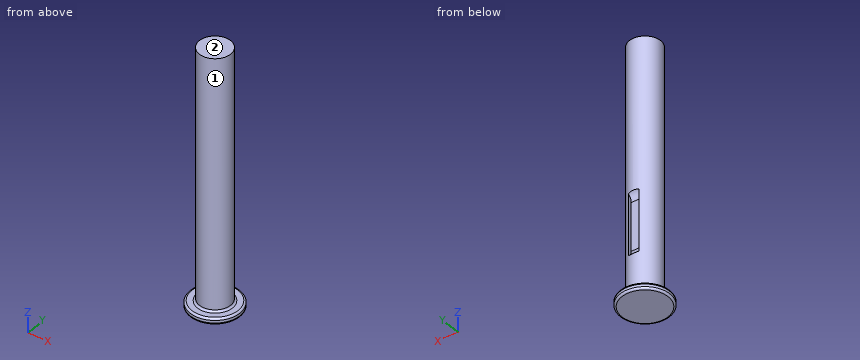
```python
from build123d import *

# Parameters (mm, degrees)
SKETCH1_R           = 8
BOSS_EXTRUDE1_DEPTH = 2
SKETCH2_R           = 5
BOSS_EXTRUDE2_DEPTH = 80
CUT_EXTRUDE1_DEPTH  = 1.75
FILLET2_R           = 0.6


with BuildPart() as part:
    # Sketch1 → Boss-Extrude1 (new body)
    with BuildSketch(Plane.XY):
        Circle(SKETCH1_R)
    extrude(amount=BOSS_EXTRUDE1_DEPTH)

    # Sketch2 → Boss-Extrude2 (add)
    with BuildSketch(Plane.XY.offset(2)):
        Circle(SKETCH2_R)
    extrude(amount=BOSS_EXTRUDE2_DEPTH)

    # Sketch4 → Cut-Extrude1 (cut, symmetric)
    with BuildSketch(Plane(origin=(0, 0, 0), x_dir=(0, 0, -1), z_dir=(1, 0, 0))):
        with BuildLine():
            Line((-34, 5), (-14, 5))
            ThreePointArc((-14, 5), (-14.921981454, 3.908349934), (-16.291287847, 3.5))
            Line((-16.291287847, 3.5), (-31.708712153, 3.5))
            ThreePointArc((-31.708712153, 3.5), (-33.078018546, 3.908349934), (-34, 5))
        make_face()
    extrude(amount=CUT_EXTRUDE1_DEPTH, both=True, mode=Mode.SUBTRACT)

    # Fillet2
    fillet2_edges = [part.edges().sort_by_distance(p)[0] for p in [
        (-8, 0, 0),
        (-8, 0, 2),
        (-5, 0, 2),
    ]]
    fillet(fillet2_edges, radius=FILLET2_R)


solid = part.part
```
Can you work these out from the model? Positions are in its coordinate system, mm. Face numbers are marked on the shaded views. A direction names the side the tool comes from. Round coordinates to 2 decimals unless told otherwise and drop trailing zeros. Loops run counter-clockwise (first coordinate to the right, second up) from the corner with the lowest first, then second, coordinate; pieces in that order, holes last. Notation, with made-up numbers: (53.25, 36) -> (100.25, 36) arc R35 cw to (100.25, 71) -> close; hole circle Ø8 at (67.25, 75). An arc over 180 degrees is marked (long way). One line per item, written item: value. Start each with the question number.
1. For the marked faces 1 and 2, which set-ups out of +Z, -Z, +X, -X, +Y, -Y let a thin tool reach every point of the face, with its end or its side?
2. If we section it at C-C, the plane z = 55: Write out the boundary of the cut face in (x, y), then the cut area to 3 significant figures.
3. For pin 1 (4 mm diameter, centred on x = 0, z = 22, fed in from +Y); pin 2 (1 mm diameter, centred on y = -3.5, z = 37, fed in from +X); pin 3 (1.3 mm diameter, centred on y = 4, z = 21.5, fed in from +X), each with a flat end and sliding along its axis, tell me the tip position at first contact or that it passes through.
4. If we section it at A-A, the plane y = 0: Write out the boundary of the cut face in (x, z), then the cut area to 3 significant figures.
5. If we section it at B-B, the plane z = 28: Write out the boundary of the cut face in (x, y).
6. If I drill on probe 1 along Z at (x, y) = (4.5, 4.75); probe 2 along X at (y, z) = (-0.25, 20); probe 3 along Y at (x, z) = (4.5, 37.5), over which ranges is the centre line in solid material (lowest first)?
Calculated:
1. face 1: +Z
1. face 2: +Z, +X, -X, +Y, -Y
2. outline: circle Ø10 at (0, 0)
2. area: 78.5 mm²
3. pin 1: stops at y = 4.68
3. pin 2: stops at x = 4
3. pin 3: stops at x = 3.71
4. outline: (-8, 0.6) arc R0.6 ccw to (-7.4, 0) -> (7.4, 0) arc R0.6 ccw to (8, 0.6) -> (8, 1.4) arc R0.6 ccw to (7.4, 2) -> (5.6, 2) arc R0.6 cw to (5, 2.6) -> (5, 82) -> (-5, 82) -> (-5, 2.6) arc R0.6 cw to (-5.6, 2) -> (-7.4, 2) arc R0.6 ccw to (-8, 1.4) -> close
4. area: 832 mm²
5. outline: (-1.75, 3.5) -> (-1.75, 4.68) arc R5 ccw (long way) to (1.75, 4.68) -> (1.75, 3.5) -> close
6. probe 1: z = 0 to 2
6. probe 2: x = -4.99 to 4.99
6. probe 3: y = -2.18 to 2.18
